The model under review builds one solid part; all positions refer to its coordinate system, in mm. A direction names the side the tool comes from. Round coordinates to 2 decimals unless told otherwise and drop trailing zeros. Order: outer loops, then holes, each group sorted by start corner. A loop starts at its lowest first (then second) coordinate and runs counter-clockwise, first axis right, second up. Notation, with made-up numbers: M 0,-13 L 47,-13 A24 ccw 47,2 Z; hole C 58,51 d6. An arc over 180 degrees is marked long. Answer as a JSON object with one key per item and string values. Group by question number.
1) For faces 4 (the flat face through (17, -1.5, -20)), 5 (the cylindrical face through (-26.65, -0.74, -20.44)), 6 (the flat face through (27.2, 0, -17.3)), list the 3-axis set-ups (+Z, -Z, +X, -X, +Y, -Y) from which the entire face can be reached by the end or side of a thin tool; tool diameter is ignored.
2) Insertion check: pin 1 Ø4 at (y, z) = (-0.5, -7.5) entering from -X; pin 2 Ø3 at (x, y) = (12, -3.5) entering from +Z; pin 3 Ø8 at (x, y) = (9.5, 4.5) entering from -Z; pin 4 Ø11 at (x, z) = (0, 0) entering from -Y. Each pin has a flat end and moves straight along its axis. Give the tip position at first contact, or say it passes through.
3) Consider section C-C, the plane y = 8. Write out the cut boundary in (x, z) (3 decimals), then the cut area to 3 significant figures.
4) The part is to be moulded in two halves that separate along Z. For faces 1 (the cylindrical face through (-26.65, 12.74, 20.44)), 2 (the cylindrical face through (-6, 1, 0)), 3 (the flat face through (0, 13.5, 7)), say which applies: +Z half, -Z half, draft (parallel to the pull), parting line (faces both ways), or undercut.
5) To check wall thickness, follow line 1 (X direction, y = 2, z = 0) (3 decimals); line 2 (Y direction, x = -21, z = -25.5); line 3 (Z direction, x = 0, y = -0.75) (3 decimals). State the ranges of each line that lie inside material, in increasing order.
6) Consider section B-B, the plane z = 0. Write out the cut boundary in (x, y) (3 decimals), then the cut area to 3 significant figures.
7) Consider section D-D, the plane z = 8. Write out the cut boundary in (x, y), then the cut area to 3 significant figures.
8) Consider section A-A, the plane x = 0. Write out the cut boundary in (y, z) (3 decimals).
```python
from build123d import *

# Parameters (mm, degrees)
SKETCH1_R           = 32.085
BOSS_EXTRUDE1_DEPTH = 12
SKETCH3_R           = 33.585
BOSS_EXTRUDE3_DEPTH = 1.5
SKETCH4_R           = 33.585
BOSS_EXTRUDE4_DEPTH = 1.5
SKETCH5_R           = 26
BOSS_EXTRUDE5_DEPTH = 10
SKETCH6_R           = 6
CUT_EXTRUDE1_DEPTH  = 25


with BuildPart() as part:
    # Sketch1 → Boss-Extrude1 (new body)
    with BuildSketch(Plane(origin=(0, 0, 0), x_dir=(1, 0, 0), z_dir=(0, 1, 0))):
        Circle(SKETCH1_R)
    extrude(amount=BOSS_EXTRUDE1_DEPTH)

    # Sketch3 → Boss-Extrude3 (add)
    with BuildSketch(Plane(origin=(0, 12, 0), x_dir=(1, 0, 0), z_dir=(0, 1, 0))):
        Circle(SKETCH3_R)
    extrude(amount=BOSS_EXTRUDE3_DEPTH)

    # Sketch4 → Boss-Extrude4 (add)
    with BuildSketch(Plane.XZ):
        Circle(SKETCH4_R)
    extrude(amount=BOSS_EXTRUDE4_DEPTH)

    # Sketch5 → Boss-Extrude5 (add)
    with BuildSketch(Plane.XZ.offset(1.5)):
        Circle(SKETCH5_R)
    extrude(amount=BOSS_EXTRUDE5_DEPTH)

    # Sketch6 → Cut-Extrude1 (cut)
    with BuildSketch(Plane(origin=(0, 13.5, 0), x_dir=(1, 0, 0), z_dir=(0, 1, 0))):
        Circle(SKETCH6_R)
    extrude(amount=-CUT_EXTRUDE1_DEPTH, mode=Mode.SUBTRACT)


solid = part.part
```
Results list:
{
 "1": {"face 4": "-Y", "face 5": "+Y, -Y", "face 6": "none"},
 "2": {"pin 1": "x = -33.13", "pin 2": "z = 23.79", "pin 3": "z = -31.61", "pin 4": "through"},
 "3": {"outline": "C 0,0 d64.17; hole C 0,0 d12", "area": "3,120 mm^2"},
 "4": {"face 1": "parting line", "face 2": "undercut", "face 3": "draft"},
 "5": {"line 1": "-32.085 to -6, 6 to 32.085", "line 2": "-1.5 to 0, 12 to 13.5", "line 3": "-33.585 to -6, 6 to 33.585"},
 "6": {"outline": "M -33.585,-1.5 L -26,-1.5 L -26,-11.5 L -6,-11.5 L -6,13.5 L -33.585,13.5 L -33.585,12 L -32.085,12 L -32.085,0 L -33.585,0 Z; M 6,-11.5 L 26,-11.5 L 26,-1.5 L 33.585,-1.5 L 33.585,0 L 32.085,0 L 32.085,12 L 33.585,12 L 33.585,13.5 L 6,13.5 Z", "area": "1,190 mm^2"},
 "7": {"outline": "M -32.62,-1.5 L -24.74,-1.5 L -24.74,-11.5 L 24.74,-11.5 L 24.74,-1.5 L 32.62,-1.5 L 32.62,0 L 31.07,0 L 31.07,12 L 32.62,12 L 32.62,13.5 L -32.62,13.5 L -32.62,12 L -31.07,12 L -31.07,0 L -32.62,0 Z", "area": "1,440 mm^2"},
 "8": {"outline": "M -11.5,-26 L -1.5,-26 L -1.5,-33.585 L 0,-33.585 L 0,-32.085 L 12,-32.085 L 12,-33.585 L 13.5,-33.585 L 13.5,-6 L -11.5,-6 Z; M -11.5,6 L 13.5,6 L 13.5,33.585 L 12,33.585 L 12,32.085 L 0,32.085 L 0,33.585 L -1.5,33.585 L -1.5,26 L -11.5,26 Z"}
}
